Geometry: final body of the model. Coordinates: model frame, mm. A direction names the side the tool comes from. Round coordinates to 2 decimals unless told otherwise and drop trailing zeros. Loops run counter-clockwise (first coordinate to the right, second up) from the corner with the lowest first, then second, coordinate; pieces in that order, holes last. Notation, with made-up numbers: M -18,65.25 L 0,65.25 A23 ccw 0,87.25 Z; hole C -14.75,-17 d10. An arc over 180 degrees is marked long. Return JSON: item names as keys, results as strings.
from build123d import *

# Parameters (mm, degrees)
F1_DEPTH = 2.38125
F3_DEPTH = 4.7635
F4_R     = 29.21
F5_DEPTH = 4.7635
F7_DEPTH = 4.7635
F8_R     = 13.97
F9_DEPTH = 4.7635


with BuildPart() as f1:
    # F0 (on Front) → F1 (new body, symmetric)
    with BuildSketch(Plane.XZ):
        Polygon((114.696875, -97.63125), (114.696875, 97.63125), (-114.696875, 97.63125), (-114.696875, -97.63125), (-109.140625, -97.63125), (-109.140625, -113.50625), (109.140625, -113.50625), (109.140625, -97.63125), align=None)
    extrude(amount=F1_DEPTH, both=True)

    # F2 (on face) → F3 (cut, through all)
    with BuildSketch(Plane.XZ.offset(2.38125)):
        with BuildLine():
            Line((25.003125, 13.88461), (25.003125, -72.23125))
            ThreePointArc((25.003125, -72.23125), (40.696544, -84.573432), (48.992014, -66.41309))
            ThreePointArc((48.992014, -66.41309), (63.103125, -43.26539), (77.214236, -66.41309))
            ThreePointArc((77.214236, -66.41309), (85.509706, -84.573432), (101.203125, -72.23125))
            Line((101.203125, -72.23125), (101.203125, 13.88461))
            ThreePointArc((101.203125, 13.88461), (97.483381, 22.864866), (88.503125, 26.58461))
            Line((88.503125, 26.58461), (37.703125, 26.58461))
            ThreePointArc((37.703125, 26.58461), (28.722869, 22.864866), (25.003125, 13.88461))
        make_face()
    extrude(amount=-F3_DEPTH, mode=Mode.SUBTRACT)

    # F4 (on face) → F5 (cut, through all)
    with BuildSketch(Plane.XZ.offset(2.38125)):
        with Locations((0, 58.89625)):
            Circle(F4_R)
    extrude(amount=-F5_DEPTH, mode=Mode.SUBTRACT)

    # F6 (on face) → F7 (cut, through all)
    with BuildSketch(Plane.XZ.offset(2.38125)):
        with BuildLine():
            ThreePointArc((-50.8, 14.2875), (-55.5625, 9.525), (-50.8, 4.7625))
            Line((-50.8, 4.7625), (0, 4.7625))
            ThreePointArc((0, 4.7625), (4.7625, 9.525), (0, 14.2875))
            Line((0, 14.2875), (-50.8, 14.2875))
        make_face()
        with BuildLine():
            Line((-67.071875, 86.51875), (-95.646875, 86.51875))
            ThreePointArc((-95.646875, 86.51875), (-100.409375, 81.75625), (-95.646875, 76.99375))
            Line((-95.646875, 76.99375), (-67.071875, 76.99375))
            ThreePointArc((-67.071875, 76.99375), (-62.309375, 81.75625), (-67.071875, 86.51875))
        make_face()
    extrude(amount=-F7_DEPTH, mode=Mode.SUBTRACT)

    # F8 (on face) → F9 (cut, through all)
    with BuildSketch(Plane.XZ.offset(2.38125)):
        with Locations((-43.939427, 36.715232)):
            Circle(F8_R)
    extrude(amount=-F9_DEPTH, mode=Mode.SUBTRACT)


solid = f1.part
Q1. Section query C-C (x = 15). Output: boundary loops of the cut face in (y, z), plus the area to 3 significant figures.
Determined:
{"outline": "M -2.38,-113.51 L 2.38,-113.51 L 2.38,33.83 L -2.38,33.83 Z; M -2.38,83.96 L 2.38,83.96 L 2.38,97.63 L -2.38,97.63 Z", "area": "767 mm^2"}
Q2. Pull-direction query (X, two-part tool) for faces 4 (the flat face through (-114.697, 0, 1)), 5 (the flat face through (-112, 0, -97.631)), 6 (the flat face through (25.003, 0, -29)); classes: pulls with the +X half, pulls with the -X half, needs draft (parallel to the pull), parting line crosses it, or undercut.
Determined:
{"face 4": "pulls with the -X half", "face 5": "needs draft", "face 6": "undercut"}
Q3. Section query B-B (x = -16.5). Output: boundary loops of the cut face in (y, z).
Determined:
{"outline": "M -2.38,-113.51 L 2.38,-113.51 L 2.38,4.76 L -2.38,4.76 Z; M -2.38,14.29 L 2.38,14.29 L 2.38,34.79 L -2.38,34.79 Z; M -2.38,83 L 2.38,83 L 2.38,97.63 L -2.38,97.63 Z"}
Q4. Pin query (flat end, axial travel): pin 1 (1.4 mm diameter, centred on x = 111, y = -1, fed in from -Z); pin 2 (1.4 mm diameter, centred on y = 0, z = -106, fed in from -X). Return the tip coordinate at first contact, or that it passes through.
Determined:
{"pin 1": "stops at z = -97.63", "pin 2": "stops at x = -109.14"}
Q5. Section query D-D (z = -78). Output: boundary loops of the cut face in (x, y), plus the area to 3 significant figures.
Determined:
{"outline": "M -114.7,-2.38 L 26.39,-2.38 L 26.39,2.38 L -114.7,2.38 Z; M 49.02,-2.38 L 77.19,-2.38 L 77.19,2.38 L 49.02,2.38 Z; M 99.82,-2.38 L 114.7,-2.38 L 114.7,2.38 L 99.82,2.38 Z", "area": "877 mm^2"}
Q6. Material intervals for L1, parallel to X at y = 0.3, z = 9; L2, parallel to X at y = -0.1, z = -0.5; L3, parallel to Z at x = -66.5, y = 1.1, sorted ascending.
Determined:
{"L1": "x = -114.7 to -55.53, 4.73 to 25, 101.2 to 114.7", "L2": "x = -114.7 to 25, 101.2 to 114.7", "L3": "z = -113.51 to 77.03, 86.48 to 97.63"}
Q7. Section query A-A (z = -9.5). Output: boundary loops of the cut face in (x, y), plus the area to 3 significant figures.
Determined:
{"outline": "M -114.7,-2.38 L 25,-2.38 L 25,2.38 L -114.7,2.38 Z; M 101.2,-2.38 L 114.7,-2.38 L 114.7,2.38 L 101.2,2.38 Z", "area": "730 mm^2"}
Q8. Reachability of faces 1 (the flat face through (101.203, 0, -30)), 2 (the flat face through (2, 0, 97.631)), 3 (the flat face through (112, 0, -97.631)) from +Z, -Z, +X, -X, +Y, -Y: full face, straight path, thin tool, end or side. Return the list, or none.
Determined:
{"face 1": "+Y, -Y", "face 2": "+Z, +X, -X, +Y, -Y", "face 3": "-Z, +X, +Y, -Y"}
